Geometry check sheet. Reference: drawing and pictorial views, mm from the part's lowest x, y, z. A direction names the side the tool comes from. Give positions to 0.01 mm unless a question says otherwise; leave off trailing zeros. Write each loop counter-clockwise with the first axis right and the second up, starting at its lowest first coordinate (ties: lowest second). Pieces come first, ordered by that corner, then holes. Notation, with made-up numbers: (-8, 70) -> (3, 70) arc R10 cw to (3, 88) -> close; hole circle Ø10 at (50.25, 82). An arc over 180 degrees is marked (long way). Return JSON: item names as keys, results as strings.
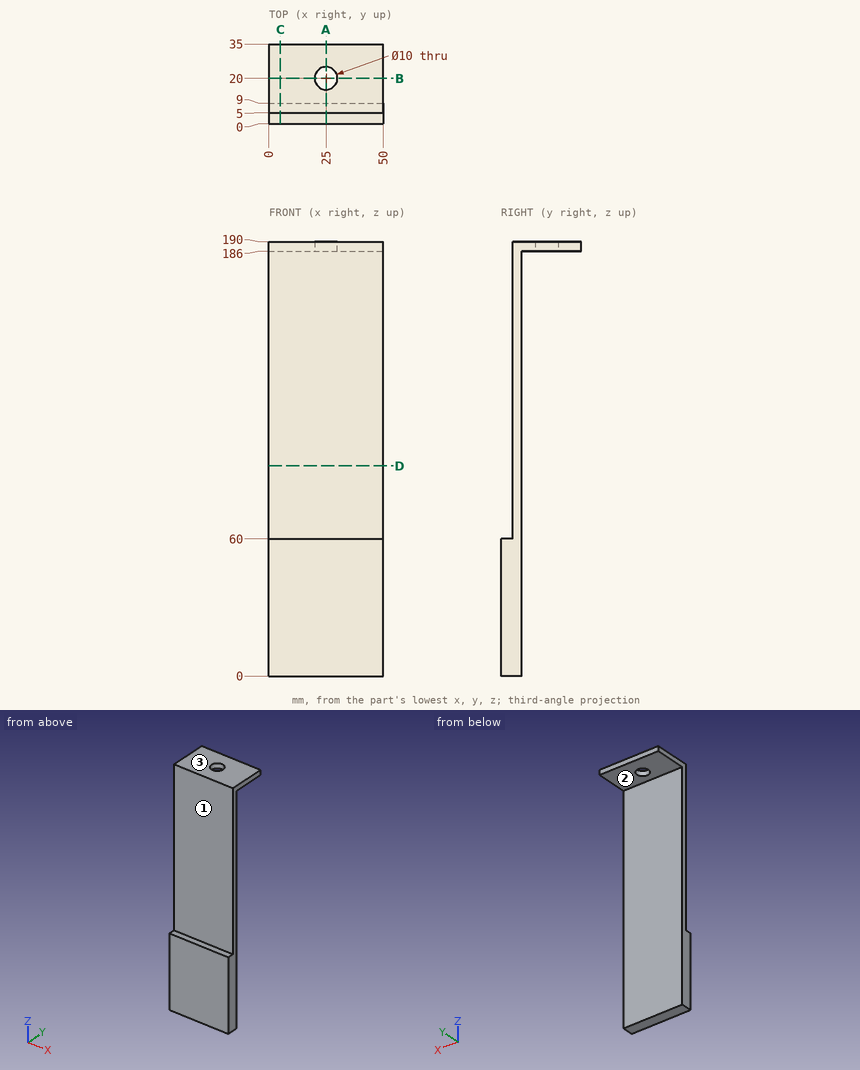
(1) Cross-section at B-B on y = 20. Enter the section's corners in (x, z).
Reply:
{"outline": "(0, 186) -> (20, 186) -> (20, 190) -> (0, 190) -> close; (30, 186) -> (50, 186) -> (50, 190) -> (30, 190) -> close"}
(2) Thickness scan on L1, parallel to Y at x = 25, z = 188; L2, parallel to Z at x = 6.5, y = 13; L3, parallel to Y at x = 45.5, z = 104. Record the ranges inside material, lowest first.
Reply:
{"L1": "5 to 15, 25 to 35", "L2": "186 to 190", "L3": "5 to 9"}
(3) Set-up check for the marked faces 1, 2 and 3: record each of +Z, -Z, +X, -X, +Y, -Y from which the full face is reachable in a straight line by a thin tool's end or side.
Reply:
{"face 1": "+Z, +X, -X, -Y", "face 2": "-Z, +X, -X, +Y", "face 3": "+Z, +X, -X, +Y, -Y"}
(4) Depth check by flat-ended pin: pin 1 Ø8 at (x, y) = (28.5, 26) entering from -Z; pin 2 Ø5.5 at (x, y) = (31.5, 3) entering from +Z; pin 3 Ø12 at (x, z) = (30.5, 34.5) entering from +Y. Enter the tip coordinate at first touch or a pass-through.
Reply:
{"pin 1": "z = 186", "pin 2": "z = 190", "pin 3": "y = 9"}
(5) Cross-section at C-C on x = 5. Enter the section's corners in (y, z), then the cut area to 3 significant figures.
Reply:
{"outline": "(0, 0) -> (9, 0) -> (9, 186) -> (35, 186) -> (35, 190) -> (5, 190) -> (5, 60) -> (0, 60) -> close", "area": "1,160 mm^2"}
(6) Cross-section at D-D on z = 92. Enter the section's corners in (x, y), then the cut area to 3 significant figures.
Reply:
{"outline": "(0, 5) -> (50, 5) -> (50, 9) -> (0, 9) -> close", "area": "200 mm^2"}
(7) Cross-section at A-A on x = 25. Enter the section's corners in (y, z), then the cut area to 3 significant figures.
Reply:
{"outline": "(0, 0) -> (9, 0) -> (9, 186) -> (15, 186) -> (15, 190) -> (5, 190) -> (5, 60) -> (0, 60) -> close; (25, 186) -> (35, 186) -> (35, 190) -> (25, 190) -> close", "area": "1,120 mm^2"}
